The model under review builds one solid part; all positions refer to its coordinate system, in mm. Give positions to 0.01 mm unless a question says otherwise; leave off trailing zeros. Loops run counter-clockwise (first coordinate to the right, second up) from the corner with the lowest first, then second, coordinate; pieces in that order, holes last. Notation, with made-up numbers: (-38.5, 27) -> (3.5, 27) arc R9 cw to (3.5, 42) -> close; hole circle Ø2 at (8.5, 73). An arc over 180 degrees is marked (long way). Write each question's results on one line, items separated by ' | '. Start each with the question number.
Q1. We need section B-B (x = 89.5). Write out the cut boundary in (y, z), plus the area to 3 significant figures.
Q2. Insertion check: pin 1 Ø0.9 at (y, z) = (1.5, -82.5) entering from -X; pin 2 Ø1.5 at (x, y) = (102, 1) entering from +Z; pin 3 Ø4 at (x, z) = (81.5, -6.5) entering from -Y; pin 4 Ø1.5 at (y, z) = (1.5, -81) entering from +X. Each pin has a flat end and moves straight along its axis. Give the tip position at first contact, or say it passes through.
Q3. We need section C-C (z = 83). Write out the cut boundary in (x, y), plus the area to 3 significant figures.
Q4. We need section A-A (z = 0). Write out the cut boundary in (x, y).
Q5. Wall thickness on L1, parallel to X at y = 1.75, z = 0; L2, parallel to X at y = 0.5, z = -26.5: over which ranges is each line inside the solid? List them lowest first. Write a range as [from, to].
from build123d import *

# Parameters (mm, degrees)
SKETCH1_W           = 200
SKETCH1_H           = 200
BOSS_EXTRUDE1_DEPTH = 3
SKETCH2_R           = 10
CUT_EXTRUDE1_DEPTH  = 10
SKETCH3_W           = 3
SKETCH3_H           = 30
SKETCH3_W_2         = 30
SKETCH3_H_2         = 3
BOSS_EXTRUDE2_DEPTH = 3


with BuildPart() as part:
    # Sketch1 → Boss-Extrude1 (new body)
    with BuildSketch(Plane(origin=(0, 0, 0), x_dir=(1, 0, 0), z_dir=(0, 1, 0))):
        Rectangle(SKETCH1_W, SKETCH1_H)
    extrude(amount=BOSS_EXTRUDE1_DEPTH)

    # Sketch2 → Cut-Extrude1 (cut)
    with BuildSketch(Plane(origin=(0, 3, 0), x_dir=(1, 0, 0), z_dir=(0, 1, 0))):
        with Locations(Location((0, 0, 0), (0, 0, 270))):
            Circle(SKETCH2_R)
    extrude(amount=-CUT_EXTRUDE1_DEPTH, mode=Mode.SUBTRACT)

    # Sketch3 → Boss-Extrude2 (add)
    with BuildSketch(Plane(origin=(0, 3, 0), x_dir=(1, 0, 0), z_dir=(0, 1, 0))):
        with Locations((101.5, 50)):
            Rectangle(SKETCH3_W, SKETCH3_H)
        with Locations((101.5, -50)):
            Rectangle(SKETCH3_W, SKETCH3_H)
        with Locations((50, -101.5)):
            Rectangle(SKETCH3_W_2, SKETCH3_H_2)
        with Locations((-50, -101.5)):
            Rectangle(SKETCH3_W_2, SKETCH3_H_2)
        with Locations((-101.5, -50)):
            Rectangle(SKETCH3_W, SKETCH3_H)
        with Locations((-101.5, 50)):
            Rectangle(SKETCH3_W, SKETCH3_H)
        with Locations((-50, 101.5)):
            Rectangle(SKETCH3_W_2, SKETCH3_H_2)
        with Locations((50, 101.5)):
            Rectangle(SKETCH3_W_2, SKETCH3_H_2)
    extrude(amount=-BOSS_EXTRUDE2_DEPTH)


solid = part.part
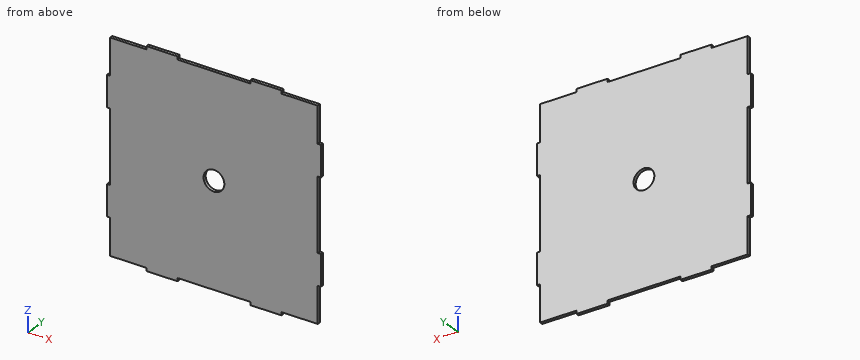
Output:
1) outline: (0, -100) -> (3, -100) -> (3, 100) -> (0, 100) -> close | area: 600 mm2
2) pin 1: x = -100 | pin 2: z = 65 | pin 3: y = 0 | pin 4: x = 100
3) outline: (-100, 0) -> (100, 0) -> (100, 3) -> (-100, 3) -> close | area: 600 mm2
4) outline: (-100, 0) -> (-10, 0) -> (-10, 3) -> (-100, 3) -> close; (10, 0) -> (100, 0) -> (100, 3) -> (10, 3) -> close
5) L1: [-100, -10], [10, 100] | L2: [-100, 100]
